Part model, mm, in its own coordinate system. Face numbers are marked on the shaded views. Coordinates: 2 decimals unless noted, no trailing zeros. Loops run counter-clockwise (first coordinate to the right, second up) from the corner with the lowest first, then second, coordinate; pieces in that order, holes last. Notation, with made-up numbers: M -16.5,-7 L -8.5,-7 A19 cw -8.5,10 Z; hole C 37,64.25 d8. An arc over 180 degrees is marked long. Answer as CSV lines item,"result". Start each with the question number.
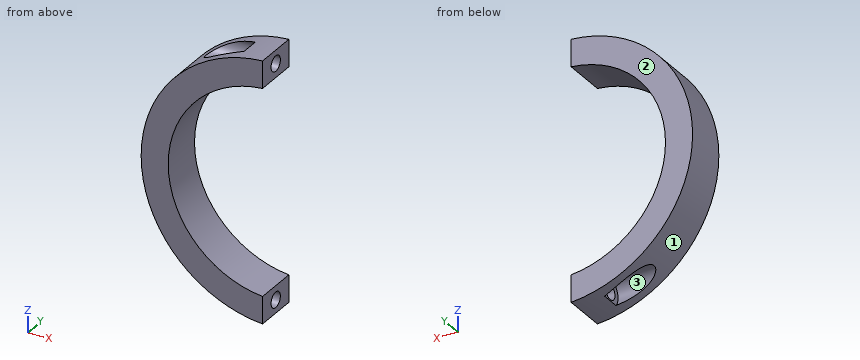
from build123d import *

# Parameters (mm, degrees)
BOSS_EXTRUDE1_DEPTH = 12.7
SKETCH2_R           = 2.25
CUT_EXTRUDE1_DEPTH  = 39.1
CUT_EXTRUDE2_START  = -10.16
SKETCH3_R           = 3.75
CUT_EXTRUDE2_DEPTH  = 28.9400001
SKETCH4_W           = 2.54
SKETCH4_H           = 76.2
CUT_EXTRUDE3_DEPTH  = 13.7000001


with BuildPart() as part:
    # Sketch1 → Boss-Extrude1 (new body)
    with BuildSketch(Plane(origin=(0, 0, 0), x_dir=(1, 0, 0), z_dir=(0, 1, 0))):
        with BuildLine():
            Line((0, 30.1625), (0, 38.1))
            ThreePointArc((0, 38.1), (-38.1, 0), (0, -38.1))
            Line((0, -38.1), (0, -30.1625))
            ThreePointArc((0, -30.1625), (-30.1625, 0), (0, 30.1625))
        make_face()
    extrude(amount=BOSS_EXTRUDE1_DEPTH)

    # Sketch2 → Cut-Extrude1 (cut, through all)
    with BuildSketch(Plane(origin=(0, 0, 0), x_dir=(0, 0, -1), z_dir=(1, 0, 0))):
        with Locations((-34.13125, 6.35)):
            Circle(SKETCH2_R)
        with Locations((34.13125, 6.35)):
            Circle(SKETCH2_R)
    extrude(amount=-CUT_EXTRUDE1_DEPTH, mode=Mode.SUBTRACT)

    # Sketch3 → Cut-Extrude2 (cut, through all)
    with BuildSketch(Plane(origin=(0, 0, 0), x_dir=(0, 0, -1), z_dir=(1, 0, 0)).offset(CUT_EXTRUDE2_START)):
        with Locations((34.13125, 6.35)):
            Circle(SKETCH3_R)
        with Locations((-34.13125, 6.35)):
            Circle(SKETCH3_R)
    extrude(amount=-CUT_EXTRUDE2_DEPTH, mode=Mode.SUBTRACT)

    # Sketch4 → Cut-Extrude3 (cut, through all)
    with BuildSketch(Plane(origin=(0, 12.7, 0), x_dir=(1, 0, 0), z_dir=(0, 1, 0))):
        with Locations((-1.27, 0)):
            Rectangle(SKETCH4_W, SKETCH4_H)
    extrude(amount=-CUT_EXTRUDE3_DEPTH, mode=Mode.SUBTRACT)


solid = part.part
Q1. Slice it at B-B, the plane x = -15. Write the cut outline in (y, z), and give its area (3 significant figures).
Q2. Two-plate mould, pull along Z, no slides. Class the marked faces 1, 2 and 3: +Z half, -Z half, draft (parallel to the pull), parting line (faces both ways), or undercut.
Q3. Flat gauge pins, fed straight in: P1, Ø7, axis at y = 6.35, z = 34.13, coming from the +X side; P2, Ø1.9, axis at y = 6, z = 32.5, coming from the -X side; P3, Ø3, axis at x = -7.5, y = 6, coming from the +Z side; P4, Ø5, axis at y = 10, z = 5.5, coming from the +X side. Where does each tip first touch, or does it go through?
Q4. Slice it at A-A, the plane y = 6.35. State how many separate pieces and enclosed holes the cut face has, and give its area (3 significant figures).
Q5. Slice it at C-C, the plane z = 0. Write the cut outline in (x, y), and give its area (3 significant figures).
Q6. Wall check: L1, parallel to Z at x = -8.5, y = 7.25; L2, parallel to Z at x = -15.5, y = 8.5; L3, parallel to Z at x = -9, y = 3.5. Give the ranges that are in metal, low to high.
Solved:
1,outline,"M 0,-35.02 L 2.71,-35.02 A3.75 cw long 9.99,-35.02 L 12.7,-35.02 L 12.7,-26.17 L 0,-26.17 Z; M 0,26.17 L 12.7,26.17 L 12.7,35.02 L 9.99,35.02 A3.75 cw long 2.71,35.02 L 0,35.02 Z"
1,area,"167 mm2"
2,face 1,"parting line"
2,face 2,"draft"
2,face 3,"undercut"
3,P1,"stops at x = -2.54"
3,P2,"stops at x = -10.16"
3,P3,"stops at z = 37.62"
3,P4,"stops at x = -29.08"
4,separate pieces,"3"
4,enclosed holes,"0"
4,area,"648 mm2"
5,outline,"M -38.1,0 L -30.16,0 L -30.16,12.7 L -38.1,12.7 Z"
5,area,"101 mm2"
6,L1,"z = -37.14 to -36.19, -32.07 to -28.94, 28.94 to 32.07, 36.19 to 37.14"
6,L2,"z = -31.06 to -25.88, 25.88 to 31.06"
6,L3,"z = -37.02 to -28.79, 28.79 to 37.02"
